Can you work these out from the model? Positions are in its coordinate system, mm. A direction names the side the tool comes from. Coordinates: 2 decimals unless noted, no trailing zeros. Loops run counter-clockwise (first coordinate to the right, second up) from the corner with the lowest first, then second, coordinate; pieces in that order, holes last.
```python
from build123d import *

# Parameters (mm, degrees)
F0_W     = 50
F0_H     = 5
F0_W_2   = 11.25
F0_H_2   = 2.25
F0_W_3   = 5
F1_DEPTH = 127


with BuildPart() as f1:
    # F0 (on Top) → F1 (new body)
    with BuildSketch(Plane.XY):
        with Locations((-25, -2.5)):
            Rectangle(F0_W, F0_H)
        Polygon((0, 25.5), (0, 0), (0, -5), (5, -5), (5, 20.5), (5, 25.5), align=None)
        Polygon((11.75, 25.5), (5, 25.5), (5, 20.5), (23, 20.5), (23, 25.5), align=None)
        with Locations((17.375, 26.625)):
            Rectangle(F0_W_2, F0_H_2)
        with Locations((25.5, 23)):
            Rectangle(F0_W_3, F0_H)
    extrude(amount=F1_DEPTH)


solid = f1.part
```
(1) If I drill on probe 1 along X at (y, z) = (-2.5, 93); probe 2 along X at (y, z) = (18.5, 96.5); probe 3 along Y at (x, z) = (-9, 70.5), over which ranges is the centre line in solid material (lowest first)?
Check values:
probe 1: x = -50 to 5
probe 2: x = 0 to 5
probe 3: y = -5 to 0
(2) I want a section at B-B on y = 16.5. Write out the boundary of the cut face in (x, z), then the cut area to 3 significant figures.
Check values:
outline: (0, 0) - (5, 0) - (5, 127) - (0, 127) - close
area: 635 mm2
(3) I want a section at C-C on x = 20. Write out the boundary of the cut face in (y, z).
Check values:
outline: (20.5, 0) - (27.75, 0) - (27.75, 127) - (20.5, 127) - close
(4) I want a section at A-A on z = 118. Write out the boundary of the cut face in (x, y).
Check values:
outline: (-50, -5) - (5, -5) - (5, 20.5) - (28, 20.5) - (28, 25.5) - (23, 25.5) - (23, 27.75) - (11.75, 27.75) - (11.75, 25.5) - (0, 25.5) - (0, 0) - (-50, 0) - close
(5) I'm going to push flat-ended pins straight in: pin 1 (2 mm diameter, centred on x = 13.5, z = 44, fed in from -Y); pin 2 (12 mm diameter, centred on y = 5, z = 98.5, fed in from +X); pin 3 (12 mm diameter, centred on x = -22.5, z = 101, fed in from +Y). Where does each tip first touch, or does it pass through?
Check values:
pin 1: stops at y = 20.5
pin 2: stops at x = 5
pin 3: stops at y = 0
(6) Which directions (+Z, -Z, +X, -X, +Y, -Y) give clear straight access to the entire face, cutting with the end or side of a thin tool? Please do faces 1 (the flat face through (25, 25.5, 63)), 2 (the flat face through (-50, -3, 63)), 3 (the flat face through (5, 8, 63)), 4 (the flat face through (-23, -5, 63)), 5 (the flat face through (6, 25.5, 63)).
Check values:
face 1: +Z, -Z, +X, +Y
face 2: +Z, -Z, -X, +Y, -Y
face 3: +Z, -Z, +X, -Y
face 4: +Z, -Z, +X, -X, -Y
face 5: +Z, -Z, -X, +Y
